Work out the finished part from the listing and answer in its coordinate system (mm). A direction names the side the tool comes from. Give positions to 0.01 mm unless a question says otherwise; leave off trailing zeros. Loops run counter-clockwise (first coordinate to the right, second up) from the corner with the lowest first, then second, coordinate; pieces in that order, holes last. Notation, with made-up numbers: (10.5, 45) - (17.5, 45) arc R21 cw to (17.5, 65) - close; hole circle Ø1 at (65.5, 50.25). An arc over 180 degrees is marked (long way). One line per item, written item: value.
from build123d import *

# Parameters (mm, degrees)
EXTRUDE_1_DEPTH     = 20
HOLE_WIZARD_2_D     = 8.2
SKETCH_7_W          = 6
SKETCH_7_H          = 6
CUT_EXTRUDE_1_DEPTH = 1.5
HOLE_WIZARD_3_D     = 3.2
HOLE_WIZARD_3_DEPTH = 7
SKETCH_11_R         = 2.5
EXTRUDE_2_DEPTH     = 10
HOLE_WIZARD_4_D     = 3.2
SKETCH_14_R         = 2.8
EXTRUDE_3_DEPTH     = 0.6
CHAMFER_1_SIZE      = 0.2
CHAMFER_1_SIZE2     = 0.072794047
HOLE_WIZARD_5_D     = 3.2


with BuildPart() as part:
    # 草图1 → 凸台-拉伸1 (new body)
    with BuildSketch(Plane.XY):
        Polygon((0, 0), (20, 0), (20, 10), (31, 10), (31, -4), (0, -4), align=None)
    extrude(amount=EXTRUDE_1_DEPTH)

    # 孔2 (through all)
    with Locations(Plane(origin=(0, 10, 0), x_dir=(1, 0, 0), z_dir=(0, 1, 0))):
        with Locations((25.5, -10)):
            Hole(HOLE_WIZARD_2_D / 2)

    # 草图7 → 切除-拉伸1 (cut, symmetric)
    with BuildSketch(Plane.XY.offset(17)):
        with Locations((25.5, 3)):
            Rectangle(SKETCH_7_W, SKETCH_7_H)
    extrude(amount=CUT_EXTRUDE_1_DEPTH, both=True, mode=Mode.SUBTRACT)

    # 孔3
    with Locations(Plane.XY.offset(20)):
        with Locations((25.5, 3)):
            Hole(HOLE_WIZARD_3_D / 2, depth=HOLE_WIZARD_3_DEPTH)

    # 草图11 → 凸台-拉伸2 (add)
    with BuildSketch(Plane.XZ.offset(4)):
        with Locations(Location((10, 10, 0), (0, 0, 180))):
            Circle(SKETCH_11_R)
    extrude(amount=EXTRUDE_2_DEPTH)

    # 孔4 (through all)
    with Locations(Plane(origin=(0, -14, 0), x_dir=(-1, 0, 0), z_dir=(0, -1, 0))):
        with Locations((-10, -10)):
            Hole(HOLE_WIZARD_4_D / 2)

    # 草图14 → 凸台-拉伸3 (add)
    with BuildSketch(Plane.XZ.offset(4)):
        with Locations(Location((10, 10, 0), (0, 0, 180))):
            Circle(SKETCH_14_R)
    extrude(amount=EXTRUDE_3_DEPTH)

    # 倒角1
    chamfer_1_edges = [part.edges().sort_by_distance(p)[0] for p in [
        (12.5, -14, 10),
    ]]
    chamfer_1_side = [part.faces().sort_by_distance(p)[0] for p in [
        (12.5, -9.3, 10),
    ]]
    chamfer(chamfer_1_edges, length=CHAMFER_1_SIZE, length2=CHAMFER_1_SIZE2, reference=chamfer_1_side[0])

    # 孔5 (through all)
    with Locations(Plane(origin=(0, 0, 0), x_dir=(1, 0, 0), z_dir=(0, 1, 0))):
        with Locations((10, -10)):
            Hole(HOLE_WIZARD_5_D / 2)


solid = part.part
1. For faces 4 (the flat face through (28.5, 3, 17)), 5 (the cylindrical face through (24.76, 1.58, 19.24)), 6 (the flat face through (20, 5, 10)), 7 (the flat face through (0, -2, 10)), determine the directions among +Z, -Z, +X, -X, +Y, -Y from which every point of the face is accessible in a straight line to the end or side of a thin tool.
Output:
face 4: none
face 5: +Z
face 6: +Z, -Z, -X, +Y
face 7: +Z, -Z, -X, +Y, -Y
2. Section A-A (x = 10) is taken. Write down the section's boundary in (y, z).
Output:
outline: (-14, 7.57) - (-13.8, 7.5) - (-4.6, 7.5) - (-4.6, 7.2) - (-4, 7.2) - (-4, 0) - (0, 0) - (0, 8.4) - (-14, 8.4) - close; (-14, 11.6) - (0, 11.6) - (0, 20) - (-4, 20) - (-4, 12.8) - (-4.6, 12.8) - (-4.6, 12.5) - (-13.8, 12.5) - (-14, 12.43) - close
3. Section C-C (y = 5.5) is taken. Write down the section's boundary in (x, z), and give its area (3 significant figures).
Output:
outline: (20, 0) - (31, 0) - (31, 20) - (20, 20) - close; hole circle Ø8.2 at (25.5, 10); hole (22.5, 15.5) - (28.5, 15.5) - (28.5, 18.5) - (22.5, 18.5) - close
area: 149 mm²
4. Find the intervals of material crossed by line 1 along Z through (x, y) = (25.5, 1); line 2 along Y through (x, z) = (25.5, 19.5); line 3 along X through (y, z) = (-4.4, 10), in increasing order.
Output:
line 1: z = 0 to 5.9, 14.1 to 15.5, 18.5 to 20
line 2: y = -4 to 1.4, 4.6 to 10
line 3: x = 7.2 to 8.4, 11.6 to 12.8
5. Section B-B (x = 25.5) is taken. Write down the section's boundary in (y, z), and give its area (3 significant figures).
Output:
outline: (-4, 0) - (10, 0) - (10, 5.9) - (-4, 5.9) - close; (-4, 14.1) - (1.4, 14.1) - (1.4, 15.5) - (0, 15.5) - (0, 18.5) - (1.4, 18.5) - (1.4, 20) - (-4, 20) - close; (4.6, 14.1) - (10, 14.1) - (10, 20) - (4.6, 20) - (4.6, 18.5) - (6, 18.5) - (6, 15.5) - (4.6, 15.5) - close
area: 138 mm²
6. Flat-ended cylindrical pins translate along their axes: pin 1 Ø1 at (x, z) = (8.5, 4.5) entering from -Y; pin 2 Ø2.5 at (y, z) = (4, 17) entering from -X; pin 3 Ø12 at (x, z) = (8, 6.5) entering from +Y. Find the tip coordinate at first contact, or state that the pin passes through.
Output:
pin 1: stops at y = -4
pin 2: stops at x = 20
pin 3: stops at y = 0
7. Section D-D (z = 17.5) is taken. Write down the section's boundary in (x, y), and give its area (3 significant figures).
Output:
outline: (0, -4) - (31, -4) - (31, 10) - (20, 10) - (20, 0) - (0, 0) - close; hole (22.5, 0) - (28.5, 0) - (28.5, 6) - (22.5, 6) - close
area: 198 mm²
8. The mould has two halves that part along Z. Classify faces 1 (the cylindrical face through (10.54, -9.14, 12.44)), 2 (the flat face through (25, 0, 17)), 3 (the flat face through (9, -14, 12)): released by +Z, released by -Z, zero draft, split by the parting line, or undercut.
Output:
face 1: split by the parting line
face 2: undercut
face 3: zero draft
